For this review, take the finished solid that the model builds, in its own axes (mm). A direction names the side the tool comes from. Coordinates: 2 decimals unless noted, no trailing zeros. Write each loop counter-clockwise with the first axis right and the second up, starting at its lowest first coordinate (ties: lowest second). Pieces come first, ordered by that corner, then holes. Notation, with made-up numbers: (89.5, -28.75) - (100.5, -28.75) arc R26 ccw to (100.5, 3.25) - close; hole circle Ø1 at (-40, 12). An arc over 180 degrees is marked (long way). Use one line per item in the form item = value. Start each with the question number.
1) Mouldability with a two-part tool opening along X and no side actions: class faces 1 (the cylindrical face through (0.09, 230.45, 17.38)), 2 (the cylindrical face through (0.08, 220.21, 13.11)), 3 (the cylindrical face through (4.44, 228.51, 55.95)) as pulls with the +X half, pulls with the -X half, needs draft (parallel to the pull), parting line crosses it, or undercut.
2) For L1, parallel to Y at x = -4, z = 46; L2, parallel to X at y = 232, z = 49 (3 decimals); L3, parallel to Z at x = -2, y = 224.25, list the stretches that pass through material, from the lowest coordinate up. Write a range as from..to.
3) Insertion check: P1, Ø1, axis at x = 3.5, z = 41.5, coming from the -Y side; P2, Ø6, axis at x = -3, z = 37.5, coming from the +Y side; P3, Ø3.5, axis at x = 0, y = 237.363, coming from the +Z side. Each pin has a flat end and moves straight along its axis. Give the tip position at first contact, or say it passes through.
4) We need section C-C (x = -2.5). Give the boundary of the cut face in (y, z) (3 decimals), plus the area to 3 significant figures.
5) Tool access review of faces 4 (the flat face through (6.35, 228, 24)), 5 (the flat face through (4, 235.331, 42)), 6 (the cylindrical face through (0.57, 235.55, 13.11)), 7 (the cylindrical face through (-0.07, 228.506, 52.994)), 8 (the flat face through (4, 221.488, 43)): name each direction out of +Z, -Z, +X, -X, +Y, -Y from which nothing blocks a thin tool from reaching the whole face with its end or side.
6) We need section A-A (y = 228). Count the separate pieces of the cut face and the enclosed holes in it, plus the area to 3 significant figures.
7) We need section B-B (z = 36). Give the boundary of the cut face in (x, y), plus the area to 3 significant figures.
Autodesk Fusion 360 part; units mm, degrees
sketch "Right" plane through (0, 0, 0) normal (1, 0, 0) x (0, 1, 0) in component "Tower"
  line L0 (0, 0) -> (0, 11.6117)
  line L1 (27.432, 9.9611) -> (27.432, 0)
  arc A0 (27.432, 9.9611) -> (25.5721, 14.4512) centre (21.082, 9.9611) ccw
  arc A1 (1.8541, 16.096) -> (0, 11.6117) centre (6.35, 11.6117) ccw
  arc A2 (5.0391, 19.281) -> (5.969, 21.526) centre (2.794, 21.526) ccw
  line L2 (5.0391, 19.281) -> (1.8541, 16.096)
  line L3 (20.7419, 19.2814) -> (25.5721, 14.4512)
  arc A3 (19.812, 21.5265) -> (20.7419, 19.2814) centre (22.987, 21.5265) ccw
  line L4 (19.812, 51.8592) -> (19.812, 21.5265)
  line L5 (19.812, 51.8592) -> (5.969, 51.8592)
  line L6 (5.969, 21.526) -> (5.969, 51.8592)
  line L7 (0, 0) -> (27.432, 0)
  circle A4 centre (12.3596, 10.3275) radius 1.8986
  line L8 (3.937, 0) -> (3.937, 12.7) construction
  line L9 (22.987, 0) -> (22.987, 12.7) construction
  circle A5 centre (12.3596, 10.3275) radius 12.7 construction
  dimension "d1" = 27.432
  dimension "d4" = 10.3275
  dimension "d5" = 6.35
  dimension "d6" = 6.8309
  dimension "d7" = 3.175
  dimension "d8" = 3.175
  dimension "d9" = 6.35
  dimension "d11" = 30.3327
  dimension "d13" = 13.843
  dimension "d14" = 9.9611
  dimension "d16" = 45
  dimension "d17" = 45
  dimension "d19" = 3.937
  dimension "d20" = 19.05
  dimension "d21" = 4.445
  dimension "d22" = 3.7973
  dimension "d23" = 12.3596
  dimension "d24" = 25.5721
  dimension "d25" = 14.4512
  dimension "d26" = 21.5265
  dimension "d28" = 12.7
  dimension "d29" = 12.7
  dimension "d46" = 16.096
  dimension "d47" = 1.8541
  dimension "d48" = 25.4
extrude "Extrude1" add sketch "Right" along normal mid plane 12.7 in component "Tower"
sketch "Front" plane through (0, 0, 0) normal (0, 1, 0) x (1, 0, 0) in component "Tower"
  line L0 (3.175, -43.9217) -> (3.175, -31.2217)
  arc A0 (3.175, -31.2217) -> (-3.175, -31.2217) centre (0, -31.2217) ccw
  line L1 (-3.175, -31.2217) -> (-3.175, -43.9217)
  arc A1 (-3.175, -43.9217) -> (3.175, -43.9217) centre (0, -43.9217) ccw
  line L2 (0, -43.9217) -> (0, -31.2217) construction
  dimension "d32" = 6.35
  dimension "d33" = 31.2217
  dimension "d34" = 12.7
  dimension "d35" = 3.175
extrude "Extrude2" cut sketch "Front" along normal up to surface (19.812 mm away) in component "Tower"
sketch "Bottom" plane through (0, 0, 0) normal (0, 0, 1) x (1, 0, 0) in component "Tower"
  circle A0 centre (0, 3.937) radius 1.8986
  circle A1 centre (0, 22.987) radius 1.8986
  dimension "d38" = 19.05
  dimension "d39" = 3.7973
  dimension "d40" = 3.7973
  dimension "d41" = 3.937
hole "Hole1" at (0, 22.987, 0) at (0, 3.937, 0) direction (0, 0, 1) diameter 3.7973 depth 14.224 tip angle 118 in component "Tower"
fillet "Fillet1" radius 6.35 2 edges at (-6.35, 12.8905, 51.8592) (6.35, 12.8905, 51.8592) in component "Tower"
component "Tower" placed x (-1, 0, 0) y (0, -1, 0) z (0, 0, 1) at (0, 241.3, 5.8979)
equation "d39 = d40"
Determined:
q1.face_1 = needs draft
q1.face_2 = undercut
q1.face_3 = pulls with the +X half
q2.L1 = 221.49..235.33
q2.L2 = -6.35..-3.175, 3.175..6.35
q2.L3 = 5.9..34.65, 52.29..57.43
q3.P1 = 221.49
q3.P2 = 235.33
q3.P3 = 26.12
q4.outline = (213.868, 5.898) - (241.3, 5.898) - (241.3, 17.51) arc R6.35 ccw to (239.446, 21.994) - (236.261, 25.179) arc R3.175 cw to (235.331, 27.424) - (235.331, 35.162) - (221.488, 35.162) - (221.488, 27.424) arc R3.175 cw to (220.558, 25.179) - (215.728, 20.349) arc R6.35 ccw to (213.868, 15.859) - close; (221.488, 51.777) - (235.331, 51.777) - (235.331, 57.245) - (221.488, 57.245) - close; hole circle Ø3.797 at (228.94, 16.225)
q4.area = 696 mm²
q5.face_4 = +Z, -Z, +X, +Y, -Y
q5.face_5 = +Z, +X, -X, +Y
q5.face_6 = -Z
q5.face_7 = +Y, -Y
q5.face_8 = +Z, +X, -X, -Y
q6.separate_pieces = 2
q6.enclosed_holes = 1
q6.area = 487 mm²
q7.outline = (-6.35, 221.49) - (-2.97, 221.49) - (-2.97, 235.33) - (-6.35, 235.33) - close; (2.97, 221.49) - (6.35, 221.49) - (6.35, 235.33) - (2.97, 235.33) - close
q7.area = 93.5 mm²
